from build123d import *

# Parameters (mm, degrees)
F0_R     = 35
F1_DEPTH = 115
F2_R     = 5
F4_DEPTH = 45


with BuildPart() as f1:
    # F0 (on Top) → F1 (new body)
    with BuildSketch(Plane.XY):
        Circle(F0_R)
    extrude(amount=F1_DEPTH)

    # F2
    f2_edges = [f1.edges().sort_by_distance(p)[0] for p in [
        (-35, 0, 115),
    ]]
    fillet(f2_edges, radius=F2_R)

    # F3 (on Front) → F4 (join)
    with BuildSketch(Plane.XZ):
        Polygon((22.900352, 83.783798), (-22.900352, 83.783798), (-22.900352, 28.148592), (-22.900352, 0), (22.900352, 0), (22.900352, 28.148592), align=None)
    extrude(amount=F4_DEPTH)


solid = f1.part
For this review, take the finished solid that the model builds, in its own axes (mm). A direction names the side the tool comes from. Coordinates: 2 decimals unless noted, no trailing zeros. Loops run counter-clockwise (first coordinate to the right, second up) from the corner with the lowest first, then second, coordinate; pieces in that order, holes last. Notation, with made-up numbers: (-28.75, 16.5) -> (26.25, 16.5) arc R4 cw to (26.25, 21.5) -> close; hole circle Ø10 at (-20, -5). An arc over 180 degrees is marked (long way). Write each question's results on one line, items separated by ' | '.
Q1. Add section A-A, the plane x = 0. State the section outline as (y, z) points, then the cut area to 3 significant figures.
Taken from the geometry:
outline: (-45, 0) -> (35, 0) -> (35, 110) arc R5 ccw to (30, 115) -> (-30, 115) arc R5 ccw to (-35, 110) -> (-35, 83.78) -> (-45, 83.78) -> close | area: 8,880 mm²
Q2. For pin 1 Ø9.5 at (y, z) = (-34, 26) entering from +X; pin 2 Ø9.5 at (y, z) = (-39.5, 46) entering from -X; pin 3 Ø5 at (x, z) = (7.5, 71.5) entering from +Y, all flat-tipped, find the tip position at first contact; note any pin that passes through.
Taken from the geometry:
pin 1: x = 22.9 | pin 2: x = -22.9 | pin 3: y = 34.64
Q3. Add section C-C, the plane z = 76. State the section outline as (x, y) points.
Taken from the geometry:
outline: (-22.9, -45) -> (22.9, -45) -> (22.9, -26.47) arc R35 ccw (long way) to (-22.9, -26.47) -> close
Q4. To check wall thickness, follow line 1 along Y through (x, z) = (18, 56); line 2 along X through (y, z) = (-38, 76.5); line 3 along X through (y, z) = (-1, 25). State the ranges of each line that lie inside material, in increasing order. Write a range as [from, to].
Taken from the geometry:
line 1: [-45, 30.02] | line 2: [-22.9, 22.9] | line 3: [-34.99, 34.99]
Q5. Add section B-B, the plane z = 99.5. State the section outline as (x, y) points.
Taken from the geometry:
outline: circle Ø70 at (0, 0)
Q6. Machinability: for faces 1 (the flat face through (0, -45, 42)), 2 (the flat face through (-22.9, -36, 42)), 3 (the flat face through (22.9, -36, 41)), which of the approach directions +Z, -Z, +X, -X, +Y, -Y give a long, thin tool a straight path to every point of the face, cutting with its end or side? Answer none if there is none.
Taken from the geometry:
face 1: +Z, -Z, +X, -X, -Y | face 2: +Z, -Z, -X, -Y | face 3: +Z, -Z, +X, -Y
